from build123d import *

# Parameters (mm, degrees)
SKETCH1_R           = 2.65
BOSS_EXTRUDE1_DEPTH = 3.75
CUT_EXTRUDE1_DEPTH  = 2.75
BOSS_EXTRUDE2_START = -3.75
BOSS_EXTRUDE2_DEPTH = 3.75


with BuildPart() as part:
    # Sketch1 → Boss-Extrude1 (new body)
    with BuildSketch(Plane(origin=(0, 0, 0), x_dir=(1, 0, 0), z_dir=(0, 1, 0))):
        with Locations(Location((0, 0, 0), (0, 0, 270))):
            Circle(SKETCH1_R)
    extrude(amount=BOSS_EXTRUDE1_DEPTH)

    # Sketch2 → Cut-Extrude1 (cut)
    with BuildSketch(Plane(origin=(0, 0, 0), x_dir=(-1, 0, 0), z_dir=(0, -1, 0))):
        Polygon((-0.749366211, 2.306312052), (-0.348066685, 2.197606558), (0, 2.425), (0.348066685, 2.197606558), (0.749366211, 2.306312052), (1.010128862, 1.982489516), (1.425379237, 1.961866211), (1.573312588, 1.573312588), (1.961866211, 1.425379237), (1.982489516, 1.010128862), (2.306312052, 0.749366211), (2.197606558, 0.348066685), (2.425, 0), (2.197606558, -0.348066685), (2.306312052, -0.749366211), (1.982489516, -1.010128862), (1.961866211, -1.425379237), (1.573312588, -1.573312588), (1.425379237, -1.961866211), (1.010128862, -1.982489516), (0.749366211, -2.306312052), (0.348066685, -2.197606558), (0, -2.425), (-0.348066685, -2.197606558), (-0.749366211, -2.306312052), (-1.010128862, -1.982489516), (-1.425379237, -1.961866211), (-1.573312588, -1.573312588), (-1.961866211, -1.425379237), (-1.982489516, -1.010128862), (-2.306312052, -0.749366211), (-2.197606558, -0.348066685), (-2.425, 0), (-2.197606558, 0.348066685), (-2.306312052, 0.749366211), (-1.982489516, 1.010128862), (-1.961866211, 1.425379237), (-1.573312588, 1.573312588), (-1.425379237, 1.961866211), (-1.010128862, 1.982489516), align=None)
    extrude(amount=-CUT_EXTRUDE1_DEPTH, mode=Mode.SUBTRACT)

    # Sketch3 → Boss-Extrude2 (add)
    with BuildSketch(Plane(origin=(0, 3.75, 0), x_dir=(1, 0, 0), z_dir=(0, 1, 0)).offset(BOSS_EXTRUDE2_START)):
        with BuildLine():
            Line((-2.649502742, 0.051334382), (-3.038574166, 0.26375564))
            ThreePointArc((-3.038574166, 0.26375564), (-3.03254237, 0.325863125), (-3.02524125, 0.387834215))
            Line((-3.02524125, 0.387834215), (-2.599921696, 0.512744745))
            ThreePointArc((-2.599921696, 0.512744745), (-2.578570239, 0.611126438), (-2.5534974, 0.708626156))
            Line((-2.5534974, 0.708626156), (-2.877518411, 1.011131938))
            ThreePointArc((-2.877518411, 1.011131938), (-2.856230611, 1.069788155), (-2.833747286, 1.127996595))
            Line((-2.833747286, 1.127996595), (-2.390725942, 1.143210159))
            ThreePointArc((-2.390725942, 1.143210159), (-2.345578748, 1.233191119), (-2.297046425, 1.321392342))
            Line((-2.297046425, 1.321392342), (-2.535657591, 1.694975097))
            ThreePointArc((-2.535657591, 1.694975097), (-2.500451378, 1.746494462), (-2.464198558, 1.7972828))
            Line((-2.464198558, 1.7972828), (-2.031312085, 1.701843475))
            ThreePointArc((-2.031312085, 1.701843475), (-1.965205918, 1.777769866), (-1.896263575, 1.851130588))
            Line((-1.896263575, 1.851130588), (-2.034472079, 2.272316738))
            ThreePointArc((-2.034472079, 2.272316738), (-1.98755959, 2.313462098), (-1.939815172, 2.353639118))
            Line((-1.939815172, 2.353639118), (-1.544263419, 2.153543706))
            ThreePointArc((-1.544263419, 2.153543706), (-1.461351973, 2.210644795), (-1.376331511, 2.264555491))
            Line((-1.376331511, 2.264555491), (-1.405453205, 2.706880361))
            ThreePointArc((-1.405453205, 2.706880361), (-1.349782122, 2.735066402), (-1.293546065, 2.762107633))
            Line((-1.293546065, 2.762107633), (-0.960183003, 2.469928866))
            ThreePointArc((-0.960183003, 2.469928866), (-0.865675909, 2.504616781), (-0.769919476, 2.535690044))
            Line((-0.769919476, 2.535690044), (-0.688124536, 2.971360736))
            ThreePointArc((-0.688124536, 2.971360736), (-0.62719288, 2.984816425), (-0.565998701, 2.997022768))
            Line((-0.565998701, 2.997022768), (-0.315770757, 2.631119311))
            ThreePointArc((-0.315770757, 2.631119311), (-0.215606244, 2.641214483), (-0.115130569, 2.647497866))
            Line((-0.115130569, 2.647497866), (0.072441528, 3.049139588))
            ThreePointArc((0.072441528, 3.049139588), (0.134805198, 3.047019455), (0.197112443, 3.043623939))
            Line((0.197112443, 3.043623939), (0.348482526, 2.626986854))
            ThreePointArc((0.348482526, 2.626986854), (0.448010755, 2.611854966), (0.546892416, 2.592953661))
            Line((0.546892416, 2.592953661), (0.828455824, 2.935329785))
            ThreePointArc((0.828455824, 2.935329785), (0.888332969, 2.917767046), (0.947838287, 2.898983025))
            Line((0.947838287, 2.898983025), (0.990839371, 2.457791151))
            ThreePointArc((0.990839371, 2.457791151), (1.08347759, 2.418382995), (1.174552138, 2.37548464))
            Line((1.174552138, 2.37548464), (1.532415194, 2.637082417))
            ThreePointArc((1.532415194, 2.637082417), (1.586043513, 2.605180603), (1.639007966, 2.572188346))
            Line((1.639007966, 2.572188346), (1.570938134, 2.134163391))
            ThreePointArc((1.570938134, 2.134163391), (1.650865543, 2.072955127), (1.72841043, 2.008755183))
            Line((1.72841043, 2.008755183), (2.140087281, 2.173137462))
            ThreePointArc((2.140087281, 2.173137462), (2.184097109, 2.128901082), (2.227192746, 2.083773613))
            Line((2.227192746, 2.083773613), (2.052329077, 1.676438296))
            ThreePointArc((2.052329077, 1.676438296), (2.114523543, 1.597275864), (2.173666338, 1.515808251))
            Line((2.173666338, 1.515808251), (2.613289814, 1.572646288))
            ThreePointArc((2.613289814, 1.572646288), (2.644915852, 1.518854876), (2.675434815, 1.464427721))
            Line((2.675434815, 1.464427721), (2.404764636, 1.113376418))
            ThreePointArc((2.404764636, 1.113376418), (2.445318252, 1.021233884), (2.482342795, 0.927617511))
            Line((2.482342795, 0.927617511), (2.922289737, 0.873339964))
            ThreePointArc((2.922289737, 0.873339964), (2.939544805, 0.813373432), (2.955569475, 0.753066449))
            Line((2.955569475, 0.753066449), (2.606099988, 0.480357004))
            ThreePointArc((2.606099988, 0.480357004), (2.622464622, 0.381024024), (2.635044526, 0.281141151))
            Line((2.635044526, 0.281141151), (3.047671448, 0.119158478))
            ThreePointArc((3.047671448, 0.119158478), (3.049471346, 0.056784744), (3.049994836, -0.005612758))
            Line((3.049994836, -0.005612758), (2.643684494, -0.182845006))
            ThreePointArc((2.643684494, -0.182845006), (2.634831895, -0.283126977), (2.622176718, -0.383000341))
            Line((2.622176718, -0.383000341), (2.981556754, -0.642510173))
            ThreePointArc((2.981556754, -0.642510173), (2.967788388, -0.703371938), (2.952777803, -0.763939294))
            Line((2.952777803, -0.763939294), (2.51515658, -0.834558193))
            ThreePointArc((2.51515658, -0.834558193), (2.48164299, -0.929488069), (2.444547903, -1.023076513))
            Line((2.444547903, -1.023076513), (2.728099883, -1.363807547))
            ThreePointArc((2.728099883, -1.363807547), (2.699628371, -1.419333175), (2.670026882, -1.474264715))
            Line((2.670026882, -1.474264715), (2.228592128, -1.433833019))
            ThreePointArc((2.228592128, -1.433833019), (2.172523329, -1.517446008), (2.113319153, -1.598869025))
            Line((2.113319153, -1.598869025), (2.303226464, -1.999411878))
            ThreePointArc((2.303226464, -1.999411878), (2.261840774, -2.046112488), (2.219508352, -2.091956662))
            Line((2.219508352, -2.091956662), (1.801997037, -1.943014843))
            ThreePointArc((1.801997037, -1.943014843), (1.726896037, -2.010057232), (1.649302788, -2.074198716))
            Line((1.649302788, -2.074198716), (1.733632855, -2.509385806))
            ThreePointArc((1.733632855, -2.509385806), (1.681933403, -2.544327028), (1.629529949, -2.578203278))
            Line((1.629529949, -2.578203278), (1.262175844, -2.330109898))
            ThreePointArc((1.262175844, -2.330109898), (1.172761516, -2.376369169), (1.081654663, -2.419198873))
            Line((1.081654663, -2.419198873), (1.055108718, -2.861685796))
            ThreePointArc((1.055108718, -2.861685796), (0.996343971, -2.882672144), (0.937162187, -2.902451901))
            Line((0.937162187, -2.902451901), (0.643047502, -2.570795579))
            ThreePointArc((0.643047502, -2.570795579), (0.544938076, -2.593365091), (0.446042198, -2.612191868))
            Line((0.446042198, -2.612191868), (0.31028822, -3.034175542))
            ThreePointArc((0.31028822, -3.034175542), (0.248150583, -3.039888368), (0.185909078, -3.044328795))
            Line((0.185909078, -3.044328795), (-0.016485881, -2.649948719))
            ThreePointArc((-0.016485881, -2.649948719), (-0.117125827, -2.647410346), (-0.217596739, -2.641051241))
            Line((-0.217596739, -2.641051241), (-0.454028829, -3.01601688))
            ThreePointArc((-0.454028829, -3.01601688), (-0.515635019, -3.006097225), (-0.577025382, -2.994919316))
            Line((-0.577025382, -2.994919316), (-0.674983394, -2.562595836))
            ThreePointArc((-0.674983394, -2.562595836), (-0.771830284, -2.535109073), (-0.867563272, -2.503963652))
            Line((-0.867563272, -2.503963652), (-1.189817576, -2.808350786))
            ThreePointArc((-1.189817576, -2.808350786), (-1.247021377, -2.783421938), (-1.303703216, -2.757328041))
            Line((-1.303703216, -2.757328041), (-1.291069219, -2.314225631))
            ThreePointArc((-1.291069219, -2.314225631), (-1.378037806, -2.263517573), (-1.463017615, -2.209542817))
            Line((-1.463017615, -2.209542817), (-1.850845709, -2.424225683))
            ThreePointArc((-1.850845709, -2.424225683), (-1.900052795, -2.385854014), (-1.948464581, -2.346483705))
            Line((-1.948464581, -2.346483705), (-1.826032417, -1.920444119))
            ThreePointArc((-1.826032417, -1.920444119), (-1.897658144, -1.84970094), (-1.96654518, -1.776288281))
            Line((-1.96654518, -1.776288281), (-2.395578399, -1.887777565))
            ThreePointArc((-2.395578399, -1.887777565), (-2.433696908, -1.838374108), (-2.470796751, -1.788201167))
            Line((-2.470796751, -1.788201167), (-2.246259282, -1.40599404))
            ThreePointArc((-2.246259282, -1.40599404), (-2.298041642, -1.319660794), (-2.346507479, -1.231423019))
            Line((-2.346507479, -1.231423019), (-2.789788088, -1.23271344))
            ThreePointArc((-2.789788088, -1.23271344), (-2.814422894, -1.175382395), (-2.837879674, -1.117559374))
            Line((-2.837879674, -1.117559374), (-2.525345415, -0.803200184))
            ThreePointArc((-2.525345415, -0.803200184), (-2.554030732, -0.706701507), (-2.579030083, -0.60918292))
            Line((-2.579030083, -0.60918292), (-3.008705131, -0.500193395))
            ThreePointArc((-3.008705131, -0.500193395), (-3.018308338, -0.438537084), (-3.02664818, -0.376697215))
            Line((-3.02664818, -0.376697215), (-2.645754808, -0.149938307))
            ThreePointArc((-2.645754808, -0.149938307), (-2.649540678, -0.049337565), (-2.649502742, 0.051334382))
        make_face()
        Polygon((0.749366211, 2.306312052), (0.348066685, 2.197606558), (0, 2.425), (-0.348066685, 2.197606558), (-0.749366211, 2.306312052), (-1.010128862, 1.982489516), (-1.425379237, 1.961866211), (-1.573312588, 1.573312588), (-1.961866211, 1.425379237), (-1.982489516, 1.010128862), (-2.306312052, 0.749366211), (-2.197606558, 0.348066685), (-2.425, 0), (-2.197606558, -0.348066685), (-2.306312052, -0.749366211), (-1.982489516, -1.010128862), (-1.961866211, -1.425379237), (-1.573312588, -1.573312588), (-1.425379237, -1.961866211), (-1.010128862, -1.982489516), (-0.749366211, -2.306312052), (-0.348066685, -2.197606558), (0, -2.425), (0.348066685, -2.197606558), (0.749366211, -2.306312052), (1.010128862, -1.982489516), (1.425379237, -1.961866211), (1.573312588, -1.573312588), (1.961866211, -1.425379237), (1.982489516, -1.010128862), (2.306312052, -0.749366211), (2.197606558, -0.348066685), (2.425, 0), (2.197606558, 0.348066685), (2.306312052, 0.749366211), (1.982489516, 1.010128862), (1.961866211, 1.425379237), (1.573312588, 1.573312588), (1.425379237, 1.961866211), (1.010128862, 1.982489516), align=None, mode=Mode.SUBTRACT)
    extrude(amount=BOSS_EXTRUDE2_DEPTH)


solid = part.part
Can you work these out from the model? Positions are in its coordinate system, mm. Give positions to 0.01 mm unless a question says otherwise; leave off trailing zeros. Use a Markdown table: item, result. Add a question column.
Item 1: We'd pull the mould along X, two halves only. Please class faces 1 (the flat face through (0, 2.75, 0)), 2 (the flat face through (0, 3.75, 0)): +X half, -X half, draft (parallel to the pull), parting line (faces both ways), or undercut.
Item 2: If I drill on L1, parallel to Y at x = -1.25, z = -0.75; L2, parallel to X at y = 1.7, z = -1.25; L3, parallel to Z at x = -1.75, y = 2, over which ranges is the centre line in solid material (lowest first)? Write a range as [from, to].
Item 3: Will this pin go through, and if not, where does the flat tip stop? pin 1 (2 mm diameter, centred on x = 1.5, y = 2.5, fed in from -Z).
Answer sheet:
| question | item | result |
|---|---|---|
| 1 | face 1 | undercut |
| 1 | face 2 | draft |
| 2 | L1 | y = [2.75, 3.75] |
| 2 | L2 | x = [-2.34, -1.97], [1.97, 2.51] |
| 2 | L3 | z = [-2.26, -1.51], [1.51, 2.37] |
| 3 | pin 1 | stops at z = -2.94 |
